Could you check a few things on this model? Use its own coordinates, in mm. A direction names the side the tool comes from. Give positions to 0.01 mm unless a question says otherwise; leave off trailing zeros. Order: outer loops, then holes, each group sorted by start corner. A loop starts at its lowest first (then second) coordinate and runs counter-clockwise, first axis right, second up. Notation, with made-up numbers: M -35,22.25 L 1,22.25 A12 cw 1,36.25 Z; hole C 73.5,-19.5 d10. An arc over 180 degrees is marked long. Use a Markdown table: item, result. Add a question column.
Item 1: I'm going to push flat-ended pins straight in: pin 1 Ø7 at (x, y) = (0, 0) entering from +Z; pin 2 Ø1.5 at (x, z) = (25.5, 2.5) entering from +Y; pin 3 Ø1 at (x, z) = (14.5, 21.5) entering from -Y. Where does each tip first touch, or does it pass through?
Item 2: Suppose I cut it at A-A on z = 23. Write out the boundary of the cut face in (x, y), plus the area to 3 significant figures.
Item 3: For faces 1 (the face through (-0.56, 46.99, 22.15)), 2 (the face through (0, 0, 5)), 3 (the face through (3.45, -26.274, 22.249)), which set-ups out of +Z, -Z, +X, -X, +Y, -Y let a thin tool reach every point of the face, with its end or its side?
Item 4: Suppose I cut it at C-C on x = 37.5. Write out the boundary of the cut face in (y, z), plus the area to 3 significant figures.
Item 5: Suppose I cut it at B-B on y = 0. Write out the boundary of the cut face in (x, z).
Item 6: If we mould it in two halves opening along Y, with no side actions, what happens to faces 4 (the face through (0.867, -3.905, 3.479)), 5 (the face through (-0.56, 46.99, 2.85)), 6 (the face through (47.15, 0.56, 3.01))? For each: released by +Y, released by -Y, zero draft, split by the parting line, or undercut.
Item 7: If I drill on L1, parallel to Z at x = -9, y = -9.5; L2, parallel to Y at x = 0, z = 23.4; L3, parallel to Y at x = 1.5, z = 9.5, over which ranges is the centre line in solid material (lowest first)? Write a range as from..to.
from build123d import *

# Parameters (mm, degrees)
SKETCH1_W           = 100
SKETCH1_H           = 100
BOSS_EXTRUDE1_DEPTH = 25
FILLET2_R           = 10
CUT_EXTRUDE1_START  = -2
SKETCH5_R           = 4
CUT_EXTRUDE1_DEPTH  = 3


with BuildPart() as part:
    # Sketch1 → Boss-Extrude1 (new body)
    with BuildSketch(Plane(origin=(0, 0, 0), x_dir=(0, 1, 0), z_dir=(0, 0, 1))):
        Rectangle(SKETCH1_W, SKETCH1_H)
    extrude(amount=BOSS_EXTRUDE1_DEPTH)

    # Sketch4 → Cut-Revolve2 (revolve, cut)
    with BuildSketch(Plane(origin=(0, 0, 0), x_dir=(0, -1, 0), z_dir=(-1, 0, 0)), mode=Mode.PRIVATE) as cut_revolve2_sk:
        with BuildLine():
            Line((0, 25), (0, 9))
            Line((0, 9), (-18.5, 9))
            ThreePointArc((-18.5, 9), (-24.269303538, 12.850991806), (-26.5, 19.41902001))
            Line((-26.5, 19.41902001), (-26.5, 25))
            Line((-26.5, 25), (0, 25))
        make_face()
    revolve(cut_revolve2_sk.sketch.rotate(Axis((0, 0, 0), (0, 0, 1)), 90), axis=Axis((0, 0, 0), (0, 0, 1)), mode=Mode.SUBTRACT)

    # Fillet2
    fillet2_edges = [part.edges().sort_by_distance(p)[0] for p in [
        (0, -50, 25),
        (50, 0, 25),
        (0, 50, 25),
        (50, 0, 0),
        (0, -50, 0),
        (-50, 0, 0),
        (0, 50, 0),
        (50, 50, 12.5),
        (50, -50, 12.5),
        (-50, -50, 12.5),
        (-50, 50, 12.5),
        (-50, 0, 25),
    ]]
    fillet(fillet2_edges, radius=FILLET2_R)

    # Sketch5 → Cut-Extrude1 (cut)
    with BuildSketch(Plane(origin=(0, 0, 0), x_dir=(1, 0, 0), z_dir=(0, 0, -1)).offset(CUT_EXTRUDE1_START)):
        with Locations(Location((0, 0, 0), (0, 0, 180))):
            Circle(SKETCH5_R)
    extrude(amount=-CUT_EXTRUDE1_DEPTH, mode=Mode.SUBTRACT)


solid = part.part
Findings below:
| question | item | result |
|---|---|---|
| 1 | pin 1 | stops at z = 9 |
| 1 | pin 2 | stops at y = 47.38 |
| 1 | pin 3 | stops at y = -48 |
| 2 | outline | M -46,-40 A6 ccw -40,-46 L 40,-46 A6 ccw 46,-40 L 46,40 A6 ccw 40,46 L -40,46 A6 ccw -46,40 Z; hole C 0,0 d53 |
| 2 | area | 6,230 mm^2 |
| 3 | face 1 | +Z, +X, -X, +Y |
| 3 | face 2 | none |
| 3 | face 3 | +Z |
| 4 | outline | M -50,10 A10 ccw -40,0 L 40,0 A10 ccw 50,10 L 50,15 A10 ccw 40,25 L -40,25 A10 ccw -50,15 Z |
| 4 | area | 2,410 mm^2 |
| 5 | outline | M -50,10 A10 ccw -40,0 L 40,0 A10 ccw 50,10 L 50,15 A10 ccw 40,25 L 26.5,25 L 26.5,19.42 A10.78 cw 18.5,9 L -18.5,9 A10.78 cw -26.5,19.42 L -26.5,25 L -40,25 A10 ccw -50,15 Z; hole M -4,2 L 4,2 L 4,5 L -4,5 Z |
| 6 | face 4 | undercut |
| 6 | face 5 | released by +Y |
| 6 | face 6 | zero draft |
| 7 | L1 | z = 0..9 |
| 7 | L2 | y = -45.43..-26.5, 26.5..45.43 |
| 7 | L3 | y = -49.99..-19.89, 19.89..49.99 |
